For this review, take the finished solid that the model builds, in its own axes (mm). A direction names the side the tool comes from. Coordinates: 2 decimals unless noted, no trailing zeros. Order: outer loops, then holes, each group sorted by start corner. A loop starts at its lowest first (then second) coordinate and runs counter-clockwise, first axis right, second up. Notation, with made-up numbers: (-8, -17) -> (44, -17) arc R22 ccw to (44, -1) -> close; hole circle Ø3 at (56, 20.5). An arc over 180 degrees is marked (long way). Return JSON: item names as keys, results as strings. Group by question number.
Item 1: Take a section at B-B (z = 47.25). Write out the cut boundary in (x, y).
Item 2: For line 1 along X through (y, z) = (-2, 45.25); line 2 along Z through (x, y) = (46.5, 94.5); line 3 along Y through (x, z) = (127.5, 50.5), list the stretches that pass through material, from the lowest coordinate up.
Item 3: Take a section at A-A (y = 10.5). Write out the cut boundary in (x, z), then the cut area to 3 significant figures.
Item 4: Take a section at D-D (x = 135). Write out the cut boundary in (y, z).
Item 5: Insertion check: pin 1 (4.5 mm diameter, centred on y = 30, z = 48.5, fed in from -X); pin 2 (4 mm diameter, centred on x = 74.5, z = 45, fed in from -Y); pin 3 (3 mm diameter, centred on y = 5.5, z = 49.5, fed in from +X). Each pin has a flat end and moves straight along its axis. Give the tip position at first contact, or say it passes through.
Item 6: Take a section at C-C (y = 71.5). Count the separate pieces of the cut face and the enclosed holes in it, then the cut area to 3 significant figures.
Item 7: Machinability: for faces 1 (the flat face through (84, 114.1, 43)), 2 (the flat face through (109, 75.5, 43)), 3 (the flat face through (87, -4.5, 44)), 4 (the flat face through (69.356, 56, 43)), 5 (the flat face through (87.611, 37, 53)), which of the approach directions +Z, -Z, +X, -X, +Y, -Y give a long, thin tool a straight path to every point of the face, cutting with its end or side? Answer none if there is none.
Item 8: Draft analysis for pull direction Y (two halves, no side actions). For faces 6 (the flat face through (169.611, 54, 43)), 7 (the flat face through (109, 2, 57.136)), 8 (the flat face through (109, 79.5, 47)), 9 (the flat face through (43.022, 56, 43)), state which applies: +Y half, -Y half, draft (parallel to the pull), parting line (faces both ways), or undercut.
```python
from build123d import *

# Parameters (mm, degrees)
SKETCH016_R            = 1.6
PAD005_DEPTH           = 4
FILLET_R               = 5
SKETCH017_W            = 35
SKETCH017_H            = 80
POCKET011_DEPTH        = 5
SKETCH018_W            = 43
SKETCH018_H            = 84
PAD006_DEPTH           = 15
SKETCH019_W            = 35
SKETCH019_H            = 15
POCKET012_DEPTH        = 80
CHAMFER002_SIZE        = 11
CHAMFER003_SIZE        = 11
SKETCH020_W            = 4
SKETCH020_H            = 2
POCKET013_DEPTH        = 135.111544
SKETCH021_W            = 3
SKETCH021_H            = 80
POCKET014_DEPTH        = 4.001
LINEARPATTERN002_COUNT = 7
LINEARPATTERN002_PITCH = 11.666667


with BuildPart() as part:
    # Sketch016 (on Face1 of ShapeBinder001) → Pad005 (new body)
    with BuildSketch(Plane.XY.offset(41.135521)):
        Polygon((-4.5, 114.100381), (-4.5, -4.5), (6.555272, -4.5), (6.555272, -10.5), (12.555272, -10.5), (12.555272, -4.5), (152.555272, -4.5), (152.555272, -10.5), (158.555272, -10.5), (158.555272, -4.5), (169.610544, -4.5), (169.610544, 114.100381), align=None)
        with Locations((9.555272, 110.350381)):
            Circle(SKETCH016_R, mode=Mode.SUBTRACT)
        with Locations((155.555272, 110.350381)):
            Circle(SKETCH016_R, mode=Mode.SUBTRACT)
        with Locations((9.555272, -7.5)):
            Circle(SKETCH016_R, mode=Mode.SUBTRACT)
        with Locations((155.555272, -7.5)):
            Circle(SKETCH016_R, mode=Mode.SUBTRACT)
    extrude(amount=PAD005_DEPTH)

    # Fillet
    fillet_edges = [part.edges().sort_by_distance(p)[0] for p in [
        (158.555272, -4.5, 43.135521),
        (152.555272, -4.5, 43.135521),
        (6.555272, -4.5, 43.135521),
        (12.555272, -4.5, 43.135521),
    ]]
    fillet(fillet_edges, radius=FILLET_R)

    # Sketch017 (on Face5 of Fillet) → Pocket011 (cut)
    with BuildSketch(Plane.XY.offset(45.135521)):
        with Locations((109.110544, 35.5)):
            Rectangle(SKETCH017_W, SKETCH017_H)
    extrude(amount=-POCKET011_DEPTH, mode=Mode.SUBTRACT)

    # Sketch018 (on Face5 of Pocket011) → Pad006 (join)
    with BuildSketch(Plane.XY.offset(45.135521)):
        with Locations((109.110544, 37.5)):
            Rectangle(SKETCH018_W, SKETCH018_H)
    extrude(amount=PAD006_DEPTH)

    # Sketch019 (on Face30 of Pad006) → Pocket012 (cut)
    with BuildSketch(Plane.XZ.offset(4.5)):
        with Locations((109.110544, 48.635521)):
            Rectangle(SKETCH019_W, SKETCH019_H)
    extrude(amount=-POCKET012_DEPTH, mode=Mode.SUBTRACT)

    # Chamfer002
    chamfer002_edges = [part.edges().sort_by_distance(p)[0] for p in [
        (109.110544, 75.5, 56.135521),
    ]]
    chamfer(chamfer002_edges, length=CHAMFER002_SIZE)

    # Chamfer003
    chamfer003_edges = [part.edges().sort_by_distance(p)[0] for p in [
        (109.110544, 79.5, 60.135521),
    ]]
    chamfer(chamfer003_edges, length=CHAMFER003_SIZE)

    # Sketch020 (on Face7 of Chamfer003) → Pocket013 (cut, through all)
    with BuildSketch(Plane.YZ.offset(130.610544)):
        with Locations((2, 56.135521)):
            Rectangle(SKETCH020_W, SKETCH020_H)
        with Locations((2, 50.135521)):
            Rectangle(SKETCH020_W, SKETCH020_H)
    extrude(amount=-POCKET013_DEPTH, mode=Mode.SUBTRACT)

    # Sketch021 (on Face4 of Pocket013) → Pocket014 (cut, through all)
    with BuildSketch(Plane.XY.offset(45.135521)):
        with Locations((9.522231, 56.277565)):
            Rectangle(SKETCH021_W, SKETCH021_H)
    pocket014 = extrude(amount=-POCKET014_DEPTH, mode=Mode.SUBTRACT)

    # LinearPattern002: Pocket014 ×7
    with Locations(*[(i * LINEARPATTERN002_PITCH, 0, 0) for i in range(1, LINEARPATTERN002_COUNT)]):
        add(pocket014, mode=Mode.SUBTRACT)


solid = part.part
```
Findings below:
{
 "1": {"outline": "(87.61, -4.5) -> (91.61, -4.5) -> (91.61, 73.39) -> (126.61, 73.39) -> (126.61, -4.5) -> (130.61, -4.5) -> (130.61, 79.5) -> (87.61, 79.5) -> close"},
 "2": {"line 1": "x = 87.61 to 91.61, 126.61 to 130.61", "line 2": "z = 41.14 to 45.14", "line 3": "y = -4.5 to 0, 4 to 78.14"},
 "3": {"outline": "(-4.5, 41.14) -> (91.61, 41.14) -> (91.61, 56.14) -> (126.61, 56.14) -> (126.61, 41.14) -> (169.61, 41.14) -> (169.61, 45.14) -> (130.61, 45.14) -> (130.61, 60.14) -> (87.61, 60.14) -> (87.61, 45.14) -> (-4.5, 45.14) -> close", "area": "816 mm2"},
 "4": {"outline": "(-4.5, 41.14) -> (114.1, 41.14) -> (114.1, 45.14) -> (-4.5, 45.14) -> close"},
 "5": {"pin 1": "stops at x = 87.61", "pin 2": "stops at y = -4.5", "pin 3": "stops at x = 130.61"},
 "6": {"separate pieces": "8", "enclosed holes": "0", "area": "848 mm2"},
 "7": {"face 1": "+Z, -Z, +X, -X, +Y", "face 2": "-Z, -Y", "face 3": "+Z, -Z, -Y", "face 4": "+Z, -Z", "face 5": "+Z, -X, +Y, -Y"},
 "8": {"face 6": "draft", "face 7": "undercut", "face 8": "+Y half", "face 9": "undercut"}
}
